Part model, mm, in its own coordinate system. A direction names the side the tool comes from. Coordinates: 2 decimals unless noted, no trailing zeros. Write each loop counter-clockwise with the first axis right and the second up, starting at its lowest first coordinate (ties: lowest second). Pieces come first, ordered by that corner, then holes. Notation, with made-up numbers: M 10,50 L 38,50 A16 ccw 38,54 Z; hole C -26.75,46 d7. An arc over 180 degrees is marked long. Use a Markdown table: item, result. Add a question column.
Q1. Slice it at B-B on y = 0.5. Count the separate pieces of the cut face and the enclosed holes in it, then the cut area to 3 significant figures.
Q2. Mould opens along Y. For faces 1 (the cylindrical face through (0.76, -6.28, 0.17)), 2 (the flat face through (0, 0.1, 4.4)), 3 (the cylindrical face through (3.57, -0.54, 2.44)), 4 (the cylindrical face through (1.65, 4.34, 1.8)) say: released by +Y, released by -Y, zero draft, split by the parting line, or undercut.
Q3. Wall check: L1, parallel to Y at x = 0.7, z = 0; L2, parallel to Y at x = 8.95, z = 0. Give the ranges that are in metal, low to high. Write a range as from..to.
Q4. Slice it at C-C on x = 7.5. Write the cut outline in (y, z).
Q5. Tool access for faces 5 (the flat face through (1, -3, 1)), 6 (the cylindrical face through (0.76, 0.17, 6.28)), 7 (the flat face through (2, -3, 3)): list every direction of +Z, -Z, +X, -X, +Y, -Y with a clear straight run to the whole face (end or side of a thin tool).
Q6. Pin check, flat tips, straight feed: pin 1 Ø4 at (x, y) = (8.5, -4.5) entering from -Z; pin 2 Ø1 at (y, z) = (-5.5, 0) entering from +X; pin 3 Ø2.5 at (y, z) = (-1, 0) entering from -X; pin 4 Ø4 at (y, z) = (1.5, -1) entering from -X. Stop position of each tip, or through.
Q7. Slice it at A-A on x = 3. Write the cut outline in (y, z), then the cut area to 3 significant figures.
from build123d import *

# Parameters (mm, degrees)
HOLE_WIZARD_M3_1_D       = 2.5
FILLET_1_R               = 1
CHAMFER_1_SIZE           = 0.2
HOLE_WIZARD_M2_1_D       = 1.6
PATTERN_CIRCULAR_1_COUNT = 4
CHAMFER_2_SIZE           = 0.2


with BuildPart() as part:
    # 草图1 → 旋转1 (revolve)
    with BuildSketch(Plane.XY):
        Polygon((11, 0), (6, 0), (6, 2.5), (1, 2.5), (1, 4), (0, 4), (0, 7), (1.5, 7), (1.5, 4.7), (2, 4.7), (2, 4), (11, 4), align=None)
    revolve(axis=Axis((11, 0, 0), (-1, 0, 0)))

    # M3 螺纹孔1 (through all)
    with Locations(Plane.ZY.offset(-6)):
        with Locations((0, 0)):
            Hole(HOLE_WIZARD_M3_1_D / 2)

    # 圆角1
    fillet_1_edges = [part.edges().sort_by_distance(p)[0] for p in [
        (11, -4, 0),
    ]]
    fillet(fillet_1_edges, radius=FILLET_1_R)

    # 倒角1
    chamfer_1_edges = [part.edges().sort_by_distance(p)[0] for p in [
        (1.5, -7, 0),
        (0, -7, 0),
        (0, -4, 0),
        (1, -2.5, 0),
    ]]
    chamfer(chamfer_1_edges, length=CHAMFER_1_SIZE)

    # M2 螺纹孔1 (through all)
    with Locations(Plane.ZY):
        with Locations((0, -5.5)):
            hole_wizard_m2_1 = Hole(HOLE_WIZARD_M2_1_D / 2)

    # 阵列(圆周)1: M2 螺纹孔1 ×4 about axis
    pattern_circular_1_axis = Axis((0, 0, 0), (1, 0, 0))
    for i in range(1, PATTERN_CIRCULAR_1_COUNT):
        add(hole_wizard_m2_1.rotate(pattern_circular_1_axis, i * 360 / PATTERN_CIRCULAR_1_COUNT), mode=Mode.SUBTRACT)

    # 倒角2
    chamfer_2_edges = [part.edges().sort_by_distance(p)[0] for p in [
        (2, -4.7, 0),
    ]]
    chamfer(chamfer_2_edges, length=CHAMFER_2_SIZE)


solid = part.part
Recorded:
| question | item | result |
|---|---|---|
| 1 | separate pieces | 4 |
| 1 | enclosed holes | 0 |
| 1 | area | 48.8 mm² |
| 2 | face 1 | undercut |
| 2 | face 2 | zero draft |
| 2 | face 3 | undercut |
| 2 | face 4 | split by the parting line |
| 3 | L1 | -7..-6.3, -4.7..-4, 4..4.7, 6.3..7 |
| 3 | L2 | -4..-1.25, 1.25..4 |
| 4 | outline | C 0,0 d8; hole C 0,0 d2.5 |
| 5 | face 5 | -X |
| 5 | face 6 | +X, -X |
| 5 | face 7 | +X |
| 6 | pin 1 | z = -3.12 |
| 6 | pin 2 | through |
| 6 | pin 3 | x = 6 |
| 6 | pin 4 | x = 1 |
| 7 | outline | C 0,0 d8; hole C 0,0 d5 |
| 7 | area | 30.6 mm² |
